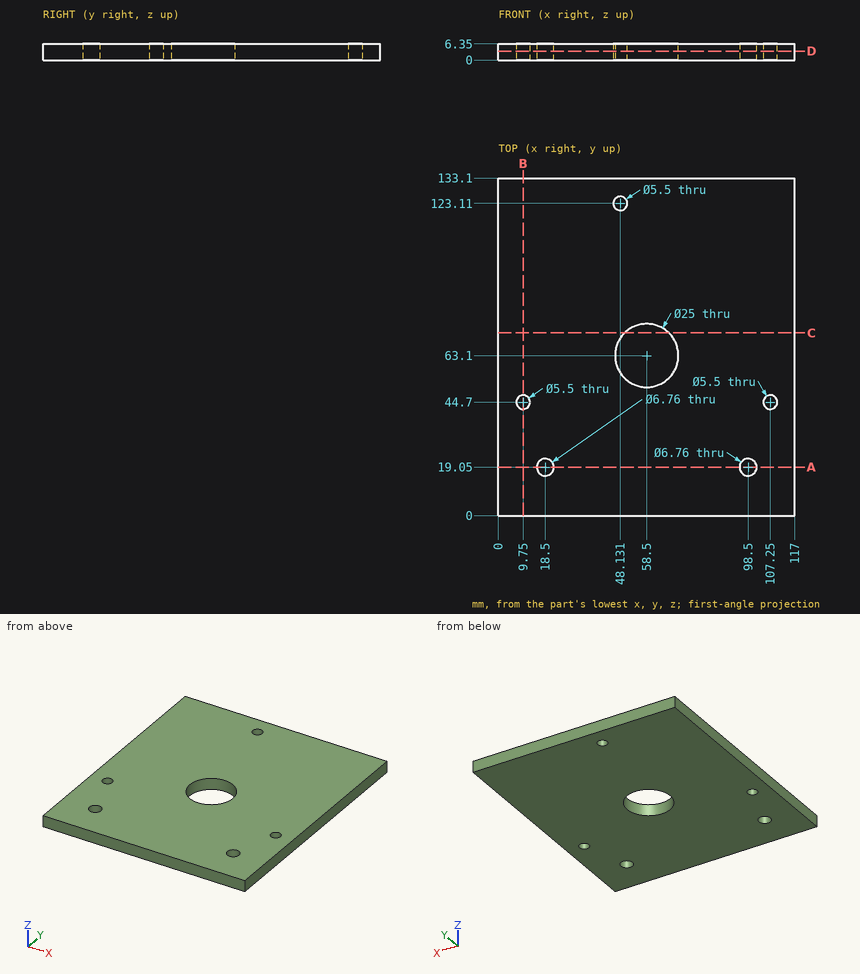
Source: three-view drawing plus pictorial views. Frame: mm from the lowest corner of the part. Give positions to 0.01 mm unless a question says otherwise; leave off trailing zeros. Write each loop counter-clockwise with the first axis right and the second up, starting at its lowest first coordinate (ties: lowest second). Pieces come first, ordered by that corner, then holes. Notation, with made-up numbers: M 14.5,47.25 L 54.5,47.25 A27 ccw 54.5,69.25 Z; hole C 19.5,-14.75 d7. An arc over 180 degrees is marked long. Use one line per item in the form item = value.
1. Ray query, L1, parallel to Y at x = 107.25, z = 3.25; L2, parallel to X at y = 63, z = 6; L3, parallel to Y at x = 7.5, z = 0.75. Return the intervals inside material, ascending.
Outcome:
L1 = 0 to 41.95, 47.45 to 133.1
L2 = 0 to 46, 71 to 117
L3 = 0 to 43.12, 46.28 to 133.1
2. Cut plane A-A on y = 19.05. Return loops of the section in (x, z), and give its area (3 significant figures).
Outcome:
outline = M 0,0 L 15.12,0 L 15.12,6.35 L 0,6.35 Z; M 21.88,0 L 95.12,0 L 95.12,6.35 L 21.88,6.35 Z; M 101.88,0 L 117,0 L 117,6.35 L 101.88,6.35 Z
area = 657 mm²
3. Cut plane D-D on z = 3.5. Return loops of the section in (x, y), and give its area (3 significant figures).
Outcome:
outline = M 0,0 L 117,0 L 117,133.1 L 0,133.1 Z; hole C 9.75,44.7 d5.5; hole C 18.5,19.05 d6.76; hole C 48.13,123.11 d5.5; hole C 58.5,63.1 d25; hole C 98.5,19.05 d6.76; hole C 107.25,44.7 d5.5
area = 14,900 mm²
4. Cut plane C-C on y = 72. Return loops of the section in (x, z).
Outcome:
outline = M 0,0 L 49.72,0 L 49.72,6.35 L 0,6.35 Z; M 67.28,0 L 117,0 L 117,6.35 L 67.28,6.35 Z
5. First-contact query: P1, Ø9, axis at x = 98.5, y = 19.05, coming from the +Z side; P2, Ø4.5, axis at x = 48.13, y = 123.11, coming from the +Z side (3 decimals). Flat tips, straight axial feed; report the tip coordinate or a pass-through.
Outcome:
P1 = 6.35
P2 = through
6. Cut plane B-B on x = 9.75. Return loops of the section in (y, z).
Outcome:
outline = M 0,0 L 41.95,0 L 41.95,6.35 L 0,6.35 Z; M 47.45,0 L 133.1,0 L 133.1,6.35 L 47.45,6.35 Z
